Autodesk Inventor part; units mm, degrees
ref_plane "YZ Plane" through (0, 0, 0) normal (1, 0, 0) x (0, 1, 0)
ref_plane "XZ Plane" through (0, 0, 0) normal (0, 1, 0) x (-1, 0, 0)
ref_plane "XY Plane" through (0, 0, 0) normal (0, 0, 1) x (1, 0, 0)
sketch "Sketch1" plane through (0, 0, 0) normal (0, 0, 1) x (1, 0, 0)
  line L0 (0, 316.484) -> (0, -316.484)
  line L1 (-541.8455, 0) -> (541.8455, 0)
  line L2 (387.0325, -226.06) -> (-387.0325, -226.06)
  line L3 (-387.0325, -226.06) -> (-387.0325, 226.06)
  line L4 (-387.0325, 226.06) -> (387.0325, 226.06)
  line L5 (387.0325, 226.06) -> (387.0325, -226.06)
  line L6 (387.0325, -226.06) -> (-387.0325, 226.06) construction
  line L7 (-387.0325, -226.06) -> (387.0325, 226.06) construction
  line L8 (368.3127, -207.3402) -> (-368.3127, -207.3402) construction
  line L9 (-368.3127, -207.3402) -> (-368.3127, 207.3402) construction
  line L10 (-368.3127, 207.3402) -> (368.3127, 207.3402) construction
  line L11 (368.3127, 207.3402) -> (368.3127, -207.3402) construction
  line L12 (368.3127, -207.3402) -> (-368.3127, 207.3402) construction
  line L13 (-368.3127, -207.3402) -> (368.3127, 207.3402) construction
  line L14 (279.4, -72.39) -> (-127, -72.39)
  line L15 (-127, -72.39) -> (-127, 226.06)
  line L16 (-127, 226.06) -> (279.4, 226.06)
  line L17 (279.4, 226.06) -> (279.4, -72.39)
  line L18 (279.4, -72.39) -> (-127, 226.06) construction
  line L19 (-127, -72.39) -> (279.4, 226.06) construction
  point P0 (0, 0)
  point P1 (-304.4952, 207.3402)
  point P2 (0, 207.3402)
  point P3 (304.4952, 207.3402)
  point P4 (-304.4952, -207.3402)
  point P5 (0, -207.3402)
  point P6 (304.4952, -207.3402)
  point P7 (-368.3127, 143.51)
  point P8 (-368.3127, -143.51)
  point P9 (368.3127, 143.51)
  point P10 (368.3127, -117.0967)
  point P11 (76.2, 76.835)
  point P12 (-209.55, 207.3402)
  dimension "d0" = 774.065
  dimension "d1" = 452.12
  dimension "d3" = 18.7198
  dimension "d4" = 18.7198
  dimension "d5" = 304.4952
  dimension "d6" = 304.4952
  dimension "d7" = 143.51
  dimension "d8" = 143.51
  dimension "d9" = 82.5373
  dimension "d10" = 82.55
  dimension "d20" = 76.2
  dimension "d23" = 406.4
  dimension "d26" = 0
  dimension "d27" = 298.45
  dimension "d28" = 82.55
  dimension "d42" = 774.065
  dimension "d43" = 452.12
extrude "Extrusion1" add sketch "Sketch1" against normal blind 6.35
hole "Hole1-M6 Clearance" at (-304.4952, 207.3402, 0) at (304.4952, 207.3402, 0) at (-304.4952, -207.3402, 0) at (0, -207.3402, 0) at (304.4952, -207.3402, 0) at (-368.3127, 143.51, 0) at (-368.3127, -143.51, 0) at (368.3127, 143.51, 0) at (368.3127, -117.0967, 0) at (-209.55, 207.3402, 0) direction (0, 0, -1) diameter 7.9375 end through all
extrude "Extrusion2" cut sketch "Sketch1" against normal up to next contours L4 L17 L1 L0 | L0 L1 L15 L4 | L1 L17 L14 L0 | L0 L14 L15 L1
sketch "Sketch3" plane through (0, 0, 0) normal (0, 0, 1) x (1, 0, 0)
  line L0 (0, 285.75) -> (0, -132.08)
  line L1 (-520.319, 0) -> (412.6865, 0)
  line L2 (-127, -72.39) -> (279.4, -72.39)
  line L3 (-387.0325, 226.06) -> (-127, 226.06)
  point P0 (0, 0)
  point P1 (-156.9974, -53.34)
  point P2 (-156.9974, -25.34)
  point P3 (-156.9974, 179.01)
  point P4 (-156.9974, 207.01)
  dimension "d29" = 28
  dimension "d30" = 28
  dimension "d31" = 156.9974
  dimension "d39" = 19.05
  dimension "d40" = 19.05
  dimension "d44" = 204.35
hole "Hole2-Tap M5" at (-156.9974, -53.34, 0) at (-156.9974, -25.34, 0) at (-156.9974, 179.01, 0) at (-156.9974, 207.01, 0) direction (0, 0, -1) diameter 4.064 end through all
fillet "Fillet1" radius 6.35 6 edges at (279.4, 226.06, -3.175) (-127, 226.06, -3.175) (-387.0325, 226.06, -3.175) (-387.0325, -226.06, -3.175) (387.0325, -226.06, -3.175) (387.0325, 226.06, -3.175)
sketch "Sketch4" plane through (0, 0, 0) normal (0, 0, 1) x (1, 0, 0)
  line L0 (0, 285.75) -> (0, -132.08)
  line L1 (-541.8455, 0) -> (541.8455, 0)
  line L2 (279.4, -72.39) -> (279.4, 219.71) construction
  line L3 (285.75, 172.085) -> (279.4, 172.085)
  line L4 (279.4, 172.085) -> (279.4, -31.115)
  line L5 (279.4, -31.115) -> (285.75, -31.115)
  line L6 (285.75, -31.115) -> (285.75, 172.085)
  line L7 (285.75, 172.085) -> (279.4, -31.115) construction
  line L8 (279.4, 172.085) -> (285.75, -31.115) construction
  line L9 (285.75, 226.06) -> (380.6825, 226.06)
  line L10 (-387.0325, 226.06) -> (387.0325, 226.06)
  line L11 (331.31, 172.085) -> (299.56, 172.085) construction
  line L12 (299.56, 172.085) -> (299.56, -31.115) construction
  line L13 (299.56, -31.115) -> (331.31, -31.115) construction
  line L14 (331.31, -31.115) -> (331.31, 172.085) construction
  line L15 (331.31, 172.085) -> (299.56, -31.115) construction
  line L16 (299.56, 172.085) -> (331.31, -31.115) construction
  circle A0 centre (316.7126, 45.085) radius 15.875
  point P0 (0, 0)
  point P1 (282.575, 70.485)
  point P2 (282.575, 70.485)
  point P3 (76.2, 76.835)
  point P4 (315.435, 70.485)
  dimension "d48" = 6.35
  dimension "d61" = 203.2
  dimension "d68" = 20.16
  dimension "d69" = 70.485
  dimension "d71" = 101.6
  dimension "d72" = 31.75
  dimension "d73" = 203.2
  dimension "d94" = 31.75
  dimension "d95" = 316.7126
  dimension "d96" = 45.085
extrude "Extrusion3" cut sketch "Sketch4" against normal up to next contours L4 L3 L6 L1 | L1 L6 L5 L4
hole "Hole3-Tap M5" at (299.56, -31.115, 0) at (299.56, 172.085, 0) at (331.31, -31.115, 0) at (331.31, 172.085, 0) direction (0, 0, -1) diameter 4.064 end through all
fillet "Fillet2" radius 3.175 4 edges at (279.4, -31.115, -3.175) (285.75, -31.115, -3.175) (285.75, 172.085, -3.175) (279.4, 172.085, -3.175)
sketch "Sketch5" plane through (0, 0, -6.35) normal (0, 0, -1) x (-1, 0, 0)
  line L0 (0, -316.484) -> (0, 316.484)
  line L1 (-541.8455, 0) -> (541.8455, 0)
  line L2 (199.898, 161.925) -> (314.198, 161.925)
  line L3 (314.198, 161.925) -> (314.198, -98.425)
  line L4 (314.198, -98.425) -> (199.898, -98.425)
  line L5 (199.898, -98.425) -> (199.898, 161.925)
  line L6 (199.898, 161.925) -> (314.198, -98.425) construction
  line L7 (314.198, 161.925) -> (199.898, -98.425) construction
  line L8 (368.3127, -207.3402) -> (368.3127, 207.3402) construction
  line L9 (387.0325, -219.71) -> (387.0325, 219.71)
  line L10 (127, 219.71) -> (127, -72.39)
  line L11 (193.548, 168.275) -> (320.548, 168.275) construction
  line L12 (320.548, 168.275) -> (320.548, -104.775) construction
  line L13 (320.548, -104.775) -> (193.548, -104.775) construction
  line L14 (193.548, -104.775) -> (193.548, 168.275) construction
  line L15 (193.548, 168.275) -> (320.548, -104.775) construction
  line L16 (320.548, 168.275) -> (193.548, -104.775) construction
  line L17 (320.548, 31.75) -> (193.548, 31.75) construction
  line L18 (193.548, 50.8) -> (320.548, 50.8) construction
  line L19 (320.548, 50.8) -> (320.548, 12.7) construction
  line L20 (320.548, 12.7) -> (193.548, 12.7) construction
  line L21 (193.548, 12.7) -> (193.548, 50.8) construction
  line L22 (193.548, 50.8) -> (320.548, 12.7) construction
  line L23 (320.548, 50.8) -> (193.548, 12.7) construction
  point P0 (0, 0)
  point P1 (257.048, 31.75)
  point P2 (304.4952, 207.3402)
  dimension "d74" = 114.3
  dimension "d75" = 260.35
  dimension "d76" = 257.048
  dimension "d77" = 31.75
  dimension "d78" = 45.4152
  dimension "d79" = 129.9845
  dimension "d80" = 130.048
  dimension "d81" = 6.35
  dimension "d82" = 6.35
  dimension "d83" = 19.05
hole "Hole4" at (-320.548, -104.775, -6.35) at (-193.548, -104.775, -6.35) at (-193.548, 12.7, -6.35) at (-193.548, 50.8, -6.35) at (-320.548, 50.8, -6.35) at (-320.548, 12.7, -6.35) at (-320.548, 168.275, -6.35) at (-193.548, 168.275, -6.35) direction (0, 0, 1) diameter 4.134 end through all
extrude "Extrusion4" cut sketch "Sketch5" against normal through all
fillet "Fillet3" radius 3.175 4 edges at (-199.898, -98.425, -3.175) (-314.198, -98.425, -3.175) (-314.198, 161.925, -3.175) (-199.898, 161.925, -3.175)
extrude "Extrusion5" cut sketch "Sketch4" against normal through all contours A0
properties material "POLYCARBONATE, CLEAR"
Work out the finished part from the listing and answer in its coordinate system (mm). Give positions to 0.01 mm unless a question says otherwise; leave off trailing zeros. Loops run counter-clockwise (first coordinate to the right, second up) from the corner with the lowest first, then second, coordinate; pieces in that order, holes last. Notation, with made-up numbers: (48.5, 48.25) -> (73.5, 48.25) arc R21 cw to (73.5, 59.25) -> close; hole circle Ø8 at (58, -17). An arc over 180 degrees is marked (long way). One line per question, with ' | ' between items. Start each with the question number.
1) Determine the mould class of faces 1 (the face through (325.2, 58.5, -3.1)), 2 (the face through (-5, -97, 0)) for opening direction Y: +Y half, -Y half, draft (parallel to the pull), parting line (faces both ways), or undercut.
2) Each of these flat-tipped pins is pushed along its axis until it touches: pin 1 (3 mm diameter, centred on x = 81.5, y = -107, fed in from +Z); pin 2 (1.9 mm diameter, centred on x = 105.5, z = -2, fed in from +Y). Where does it stop, or does it pass through?
3) Section A-A, the plane y = 192 is taken. Determine the outline of the cut face in (x, z).
4) Straight lines are drawn through the part: L1, parallel to X at y = 113, z = -2.5; L2, parallel to X at y = -50, z = -2.75; L3, parallel to Y at x = 299.56, z = -4. For each, find the intervals that lie inside material, in ascending order.
5) Section B-B, the plane z = -1.25 is taken. State how many separate pieces and enclosed holes the cut face has, then the cut area to 3 significant figures.
Resolved:
1) face 1: undercut | face 2: draft
2) pin 1: z = 0 | pin 2: y = -72.39
3) outline: (-387.03, -6.35) -> (-127, -6.35) -> (-127, 0) -> (-387.03, 0) -> close; (279.4, -6.35) -> (387.03, -6.35) -> (387.03, 0) -> (279.4, 0) -> close
4) L1: -387.03 to -314.2, -199.9 to -127, 285.75 to 387.03 | L2: -387.03 to -314.2, -199.9 to -127, 279.4 to 387.03 | L3: -226.06 to -33.15, -29.08 to 170.05, 174.12 to 226.06
5) separate pieces: 1 | enclosed holes: 28 | area: 196,000 mm2
